The listing builds one solid part. Answer for the finished solid, in the listing's coordinates (mm). Round coordinates to 2 decimals unless told otherwise and drop trailing zeros. Loops run counter-clockwise (first coordinate to the right, second up) from the corner with the lowest first, then second, coordinate; pieces in that order, holes last. Notation, with made-up numbers: (-37, 88) -> (-17, 88) arc R12 ccw to (-17, 111) -> close; hole circle Ø5 at (-0.75, -17). An arc over 180 degrees is marked (long way). Use a Markdown table: item, result. Add a question column.
Q1. Section A-A on z = 28 is taken. Give the vertices of the cut face in (x, y).
Q2. Consider line 1 (X direction, y = -0.15, z = 8); line 2 (X direction, y = -1.85, z = 16.5); line 3 (Z direction, x = -1.5, y = 2.5). Determine where each line is inside the solid, lowest interval first.
Q3. Given pin 1 Ø1 at (y, z) = (2, 6.5) entering from +X; pin 2 Ø1.5 at (y, z) = (2.5, 38) entering from +X; pin 3 Ø1.5 at (x, z) = (1.5, 38.5) entering from -Y, each flat-ended and moving along its own axis, determine where each tip first touches the part or whether it passes through.
Autodesk Inventor part; units mm, degrees
ref_plane "YZ Plane" through (0, 0, 0) normal (1, 0, 0) x (0, 1, 0)
ref_plane "XZ Plane" through (0, 0, 0) normal (0, 1, 0) x (-1, 0, 0)
ref_plane "XY Plane" through (0, 0, 0) normal (0, 0, 1) x (1, 0, 0)
sketch "Эскиз1" plane through (0, 0, 0) normal (0, 0, 1) x (1, 0, 0)
  circle A0 centre (0, 0) radius 3
  dimension "d0" = 6
extrude "Выдавливание1" add sketch "Эскиз1" along normal blind 45
chamfer "Фаска1" distance 0.5 angle 45 1 edges at (-3, 0, 45)
chamfer "Фаска2" distance 0.5 angle 45 1 edges at (-3, 0, 0)
properties part number "Штрифт" material "Сталь, углеродистая"
Checked values:
| question | item | result |
|---|---|---|
| 1 | outline | circle Ø6 at (0, 0) |
| 2 | line 1 | x = -3 to 3 |
| 2 | line 2 | x = -2.36 to 2.36 |
| 2 | line 3 | z = 0.42 to 44.58 |
| 3 | pin 1 | stops at x = 2.6 |
| 3 | pin 2 | stops at x = 2.44 |
| 3 | pin 3 | stops at y = -2.9 |
